Autodesk Inventor part; units mm, degrees
ref_plane "YZ Plane" through (0, 0, 0) normal (1, 0, 0) x (0, 1, 0)
ref_plane "XZ Plane" through (0, 0, 0) normal (0, 1, 0) x (-1, 0, 0)
ref_plane "XY Plane" through (0, 0, 0) normal (0, 0, 1) x (1, 0, 0)
sketch "Sketch1" plane through (0, 0, 0) normal (0, 1, 0) x (-1, 0, 0)
  point P0 (0, 0)
sketch "Sketch2" plane through (0, 0, 0) normal (0, 1, 0) x (-1, 0, 0)
  line L0 (0, 0) -> (38.1, 0)
  line L1 (38.1, 0) -> (38.1, -84.0465)
  arc A0 (50.8, -121.2155) -> (0, -85.725) centre (0, -139.827) ccw
  line L2 (38.1, -84.0465) -> (38.1, -101.4159)
  arc A1 (50.8, -146.6155) -> (0, -111.125) centre (0, -165.227) ccw
  line L3 (50.8, -121.2155) -> (50.8, -146.6155)
  line L4 (0, 0) -> (0, -111.125)
sketch "Sketch3" plane through (0, 0, 0) normal (0, 1, 0) x (-1, 0, 0)
  point P0 (0, 0)
  point P1 (0, 0)
  point P2 (16.5768, 0)
  point P3 (25.4, 0)
  point P4 (0, 0)
  dimension "d10" = 25.4
extrude "Extrusion1" add sketch "Sketch2" along normal blind 6.35
sketch "Sketch4" plane through (0, 6.35, 0) normal (0, 1, 0) x (1, 0, 0)
  arc A0 (-50.8, 121.2155) -> (-38.1, 101.4159) centre (0, 139.827) ccw
  arc A1 (-50.8, 146.6155) -> (0, 111.125) centre (0, 165.227) ccw
  line L0 (-50.8, 146.6155) -> (-50.8, 121.2155)
  line L1 (-50.8, 121.2155) -> (-50.8, 146.6155)
  line L2 (0, 111.125) -> (0, 92.3126)
  line L3 (0, 0) -> (0, 111.125)
  arc A2 (-42.5277, 131.7842) -> (0, 111.125) centre (0, 165.227) ccw
  arc A3 (-50.8, 121.2155) -> (0, 92.3126) centre (-9.952, 133.9155) ccw
  arc A4 (-50.8, 146.6155) -> (-44.1205, 133.9155) centre (0, 165.227) ccw
  arc A5 (-50.8, 146.6155) -> (0, 111.125) centre (0, 165.227) ccw
  point P0 (-40.6454, 104.1202)
extrude "Extrusion2" add sketch "Sketch4" along normal blind 7.62 contours L0 A1 L2 A3 A0
mirror "Mirror1" about plane through (0, 0, 0) normal (1, 0, 0) of "Extrusion1", "Extrusion2"
sketch "Sketch5" plane through (0, 6.35, 0) normal (0, 1, 0) x (1, 0, 0)
  arc A0 (38.1, 101.4159) -> (50.8, 121.2155) centre (0, 139.827) ccw
  arc A1 (-38.1, 101.4159) -> (38.1, 101.4159) centre (0, 137.2023) ccw
  line L0 (-38.1, 101.4159) -> (-38.1, 0)
  arc A2 (-38.1, 101.4159) -> (38.1, 101.4159) centre (0, 209.31) ccw
  point P0 (0, 0)
extrude "Extrusion3" add sketch "Sketch5" along normal blind 7.62
mirror "Mirror2" about plane through (0, 0, 0) normal (0, 1, 0) of "Extrusion1", "Extrusion2", "Mirror1", "Extrusion3"
sketch "Sketch6" plane through (0, 6.35, 0) normal (0, 1, 0) x (1, 0, 0)
  line L0 (-38.1, 101.4159) -> (-38.1, 0)
  line L1 (38.1, 101.4159) -> (38.1, 0)
  line L2 (-38.1, -38.1) -> (38.1, -38.1)
  line L3 (38.1, -38.1) -> (38.1, 38.1)
  line L4 (38.1, 38.1) -> (-38.1, 38.1)
  line L5 (-38.1, 38.1) -> (-38.1, -38.1)
  point P0 (0, 0)
  point P1 (-38.1, -101.4159)
  point P2 (-38.1, 38.1)
  point P3 (38.1, -101.4159)
  point P4 (-38.1, 0)
  dimension "d17" = 38.1
  dimension "d18" = 38.1
extrude "Extrusion4" cut sketch "Sketch6" against normal through all
sketch "Sketch7" plane through (0, -6.35, -137.2023) normal (0, -1, 0) x (1, 0, 0)
  point P0 (0, 137.2023)
sketch "Sketch8" plane through (-38.1, 6.35, -38.1) normal (0, 0, 1) x (1, 0, 0)
  line L0 (0, 0) -> (76.2, 0)
  line L1 (76.2, -12.7) -> (76.2, -20.32)
  line L2 (0, 0) -> (76.2, 0)
  line L3 (76.2, 0) -> (76.2, -12.7)
  line L4 (76.2, -12.7) -> (0, -12.7)
  line L5 (0, -12.7) -> (0, 0)
  point P0 (38.1, -6.35)
extrude "Extrusion5" cut sketch "Sketch8" against normal blind 12.7
sketch "Sketch9" plane through (-38.1, 6.35, -50.8) normal (0, 0, 1) x (1, 0, 0)
  line L0 (0, 0) -> (76.2, 0)
  line L1 (76.2, 0) -> (76.2, -12.7)
  line L2 (0, 0) -> (76.2, 0)
  line L3 (76.2, 0) -> (76.2, -12.7)
  line L4 (76.2, -12.7) -> (0, -12.7)
  line L5 (0, -12.7) -> (0, 0)
  point P0 (38.1, -6.35)
extrude "Extrusion6" cut sketch "Sketch9" against normal blind 25.4
sketch "Sketch10" plane through (38.1, -6.35, -101.4159) normal (1, 0, 0) x (0, 0, -1)
  point P0 (-101.4159, 6.35)
sketch "Sketch11" plane through (-38.1, 6.35, -76.2) normal (0, 0, 1) x (1, 0, 0)
  line L0 (0, -12.7) -> (-2.5454, -12.7)
  line L1 (76.2, 0) -> (76.2, -12.7)
  line L2 (0, -12.7) -> (76.2, -12.7)
  line L3 (76.2, -12.7) -> (76.2, 0)
  line L4 (76.2, 0) -> (0, 0)
  line L5 (0, 0) -> (0, -12.7)
  point P0 (38.1, -6.35)
extrude "Extrusion7" add sketch "Sketch11" along normal blind 19.05
mirror "Mirror4" about plane through (0, 0, -57.15) normal (0, 0, 1)
sketch "Sketch12" plane through (0, 13.97, 50.927) normal (0, 1, 0) x (1, 0, 0)
  point P0 (0, 50.927)
properties part number "dc motor holder 2" material "Iron, Ductile"
Geometry check sheet. Reference: the model listing, model coordinates, mm. A direction names the side the tool comes from. Give positions to 0.01 mm unless a question says otherwise; leave off trailing zeros. Write each loop counter-clockwise with the first axis right and the second up, starting at its lowest first coordinate (ties: lowest second). Pieces come first, ordered by that corner, then holes. Notation, with made-up numbers: (-9.5, 6.25) - (40.5, 6.25) arc R10 ccw to (40.5, 10.25) - close; hole circle Ø9 at (80, 89). An arc over 180 degrees is marked (long way). Use a Markdown table: item, result.
Q1. Thickness scan on L1, parallel to X at y = -4.25, z = -101; L2, parallel to Y at x = 30.5, z = -32; L3, parallel to Z at x = 29.5, y = 12.75. Record the ranges inside material, lowest first. Write a range as [from, to].
Computed:
| item | result |
|---|---|
| L1 | x = [-38.1, 38.1] |
| L2 | y = [-6.35, 6.35] |
| L3 | z = [-119.88, -94.05], [-20.25, 5.58] |
Q2. Section check B-B, the plane z = -115. Enter the section's corners in (x, y).
Computed:
| item | result |
|---|---|
| outline | (-48.07, -13.97) - (-20.11, -13.97) - (-20.11, 13.97) - (-48.07, 13.97) - (-48.07, -6.35) - close; (20.11, -13.97) - (48.07, -13.97) - (48.07, 6.35) - (48.07, 13.97) - (20.11, 13.97) - close |
Q3. Draft check along Z on faces 5 (the face through (0.598, 10.107, -84.935)), 6 (the face through (-46.586, -10.107, -112.317)), 7 (the face through (1, 13.97, -5)). Enter one of: pulls with the +Z half, pulls with the -Z half, needs draft (parallel to the pull), parting line crosses it, or undercut.
Computed:
| item | result |
|---|---|
| face 5 | undercut |
| face 6 | undercut |
| face 7 | needs draft |
Q4. Section check C-C, the plane x = -43.5. Enter the section's corners in (y, z), then the cut area to 3 significant figures.
Computed:
| item | result |
|---|---|
| outline | (-13.97, -133.06) - (13.97, -133.06) - (13.97, -107.66) - (-6.35, -107.66) - (-13.97, -107.66) - close; (-13.97, -6.64) - (6.35, -6.64) - (13.97, -6.64) - (13.97, 18.76) - (-13.97, 18.76) - close |
| area | 1,420 mm² |
Q5. Go/stop test with flat-tipped pins: P1, Ø1, axis at y = 0, z = -54.5, coming from the -X side; P2, Ø1, axis at x = 30, y = 0, coming from the -Z side; P3, Ø12, axis at y = 9.5, z = -103.5, coming from the +X side. Record where each tip stops, or that it passes through.
Computed:
| item | result |
|---|---|
| P1 | stops at x = -38.1 |
| P2 | stops at z = -120.54 |
| P3 | stops at x = 44.8 |
Q6. Section check A-A, the plane y = -12. Enter the section's corners in (x, z) (1 decimal).
Computed:
| item | result |
|---|---|
| outline | (-50.8, -146.6) arc R54.1 cw to (0, -111.1) arc R54.1 cw to (50.8, -146.6) - (50.8, -121.2) arc R54.1 ccw to (40.6, -104.1) arc R42.8 ccw to (37.5, -101.2) arc R114.4 cw to (38.1, -101.4) arc R52.3 ccw to (-38.1, -101.4) arc R114.4 cw to (-37.5, -101.2) arc R42.8 ccw to (-40.6, -104.1) arc R54.1 ccw to (-50.8, -121.2) - close; (-50.8, 6.9) arc R54.1 ccw to (-40.6, -10.2) arc R42.8 ccw to (-37.5, -13.1) arc R114.4 cw to (-38.1, -12.9) arc R52.3 ccw to (38.1, -12.9) arc R114.4 cw to (37.5, -13.1) arc R42.8 ccw to (40.6, -10.2) arc R54.1 ccw to (50.8, 6.9) - (50.8, 32.3) arc R54.1 cw to (0, -3.2) arc R54.1 cw to (-50.8, 32.3) - close |
Q7. Set-up check for faces 1 (the face through (-0.598, 10.107, -29.365)), 2 (the face through (46.443, -10.107, -112.077)), 3 (the face through (-46.443, -10.107, -2.223)), 4 (the face through (1, -13.97, -109)): record each of +Z, -Z, +X, -X, +Y, -Y from which the full face is reachable in a straight line by a thin tool's end or side.
Computed:
| item | result |
|---|---|
| face 1 | +Y |
| face 2 | +X, +Y, -Y |
| face 3 | -X, +Y, -Y |
| face 4 | +Z, -Z, +X, -X, -Y |
Q8. Section check D-D, the plane z = -96. Enter the section's corners in (x, y), then the cut area to 3 significant figures.
Computed:
| item | result |
|---|---|
| outline | (-38.1, -6.35) - (-32.17, -6.35) - (-32.17, -13.97) - (32.17, -13.97) - (32.17, -6.35) - (38.1, -6.35) - (38.1, 6.35) - (32.17, 6.35) - (32.17, 13.97) - (-32.17, 13.97) - (-32.17, 6.35) - (-38.1, 6.35) - close |
| area | 1,950 mm² |
